```python
from build123d import *

# Parameters (mm, degrees)
ESQUISSE1_R                  = 20
BOSS_EXTRU_1_DEPTH           = 25
ENL_V_MAT_EXTRU_1_REACH      = 39.749
R_P_TITION_CIRCULAIRE1_COUNT = 15
ENL_V_MAT_EXTRU_2_REACH      = 39.747
ESQUISSE5_R                  = 7.5


with BuildPart() as part:
    # Esquisse1 → Boss.-Extru.1 (new body)
    with BuildSketch(Plane(origin=(0, 0, 0), x_dir=(1, 0, 0), z_dir=(0, 1, 0))):
        with Locations(Location((0, 0, 0), (0, 0, 270))):
            Circle(ESQUISSE1_R)
    extrude(amount=BOSS_EXTRU_1_DEPTH)

    # Esquisse3 → Enlèv. mat.-Extru.1 (cut, up to next)
    with BuildSketch(Plane(origin=(0, 25, 0), x_dir=(1, 0, 0), z_dir=(0, 1, 0)), mode=Mode.PRIVATE) as enl_v_mat_extru_1_sk1:
        with BuildLine():
            ThreePointArc((2.80685469, 19.802059659), (0, 20), (-2.80685469, 19.802059659))
            Line((-2.80685469, 19.802059659), (-2.015422429, 16.848394249))
            ThreePointArc((-2.015422429, 16.848394249), (-1.276557591, 15.640396711), (0, 15.027550875))
            ThreePointArc((0, 15.027550875), (1.276557591, 15.640396711), (2.015422429, 16.848394249))
            Line((2.015422429, 16.848394249), (2.80685469, 19.802059659))
        make_face()
    enl_v_mat_extru_1_tool1 = extrude(enl_v_mat_extru_1_sk1.sketch, amount=-ENL_V_MAT_EXTRU_1_REACH, mode=Mode.PRIVATE) & part.part
    enl_v_mat_extru_1 = enl_v_mat_extru_1_tool1.solids().sort_by_distance((0, 25, -17.875874))[0]
    add(enl_v_mat_extru_1, mode=Mode.SUBTRACT)

    # Répétition circulaire1: Enlèv. mat.-Extru.1 ×15 about axis
    r_p_tition_circulaire1_axis = Axis((0, 0, 0.291044728), (0, 1, 0))
    for i in range(1, R_P_TITION_CIRCULAIRE1_COUNT):
        add(enl_v_mat_extru_1.rotate(r_p_tition_circulaire1_axis, i * 360 / R_P_TITION_CIRCULAIRE1_COUNT), mode=Mode.SUBTRACT)

    # Esquisse5 → Enlèv. mat.-Extru.2 (cut, up to next)
    with BuildSketch(Plane(origin=(0, 25, 0), x_dir=(1, 0, 0), z_dir=(0, 1, 0)), mode=Mode.PRIVATE) as enl_v_mat_extru_2_sk1:
        with Locations(Location((0, 0, 0), (0, 0, 270))):
            Circle(ESQUISSE5_R)
    enl_v_mat_extru_2_tool1 = extrude(enl_v_mat_extru_2_sk1.sketch, amount=-ENL_V_MAT_EXTRU_2_REACH, mode=Mode.PRIVATE) & part.part
    add(enl_v_mat_extru_2_tool1.solids().sort_by_distance((0, 25, 0))[0], mode=Mode.SUBTRACT)


solid = part.part
```
Read the model definition and answer for the solid it produces. Units are mm, in the model's axes. A direction names the side the tool comes from. Coordinates: 2 decimals unless noted, no trailing zeros. Write each loop counter-clockwise with the first axis right and the second up, starting at its lowest first coordinate (ties: lowest second). Pieces come first, ordered by that corner, then holes. Notation, with made-up numbers: (-20, -3) -> (-16, -3) arc R15 cw to (-16, 18) -> close; hole circle Ø7 at (68, -22.5). An arc over 180 degrees is marked (long way). Answer as a JSON object with one key per item and string values.
Q1. The part is cut by section A-A on x = -4.5. Give the vertices of the cut face in (y, z).
The answers:
{"outline": "(0, -19.49) -> (25, -19.49) -> (25, -6) -> (0, -6) -> close; (0, 6) -> (25, 6) -> (25, 15.57) -> (0, 15.57) -> close"}
Q2. Flat-ended cylindrical pins translate along their axes: pin 1 Ø2 at (y, z) = (11.5, 13.5) entering from +X; pin 2 Ø10 at (y, z) = (18, 8) entering from -X; pin 3 Ø6 at (y, z) = (15.5, 15.5) entering from -X. Find the tip coordinate at first contact, or state that the pin passes through.
The answers:
{"pin 1": "stops at x = 15.61", "pin 2": "stops at x = -19.35", "pin 3": "stops at x = -15.61"}
Q3. Consider line 1 (Z direction, x = 15.5, y = 6); line 2 (Z direction, x = 18, y = 21); line 3 (Z direction, x = 16, y = 21.25). Determine where each line is inside the solid, lowest interval first. Write a range as [from, to].
The answers:
{"line 1": "z = [-10.4, -6.8], [-3.45, 1.27], [2.88, 7.05], [12.27, 12.64]", "line 2": "z = [-8.72, -8.43], [-3.14, -0.04], [4.53, 7.69]", "line 3": "z = [-10.66, -7.13], [-3.21, 0.67], [3.56, 7.16]"}
Q4. Determine the mould class of faces 6 (the cylindrical face through (-12, 12, -16)), 7 (the cylindrical face through (0, 12, 20)), 8 (the cylindrical face through (-12.71, 12.68, -9.42)) for opening direction X: pulls with the +X half, pulls with the -X half, needs draft (parallel to the pull), parting line crosses it, or undercut.
The answers:
{"face 6": "pulls with the -X half", "face 7": "parting line crosses it", "face 8": "undercut"}
Q5. The part is cut by section B-B on x = 4. Give the vertices of the cut face in (y, z), then the cut area to 3 significant figures.
The answers:
{"outline": "(0, -19.6) -> (25, -19.6) -> (25, -6.34) -> (0, -6.34) -> close; (0, 6.34) -> (25, 6.34) -> (25, 15.37) -> (0, 15.37) -> close", "area": "557 mm2"}
Q6. A tool of negligible diameter and unlimited length cuts with its end or side. For faces 1 (the flat face through (-17.115, 12.675, 7.454)), 2 (the flat face through (-15.409, 12.675, -10.354)), 3 (the flat face through (-18.111, 12.675, 4.577)), 4 (the cylindrical face through (15.993, 12.675, 0.673)), 5 (the cylindrical face through (-8.327, 12.675, 13.95)), from which of +Z, -Z, +X, -X, +Y, -Y can it reach the whole face along a straight path? Write none if from no direction.
The answers:
{"face 1": "+Z, +Y, -Y", "face 2": "-Z, +Y, -Y", "face 3": "-X, +Y, -Y", "face 4": "+X, +Y, -Y", "face 5": "+Y, -Y"}
